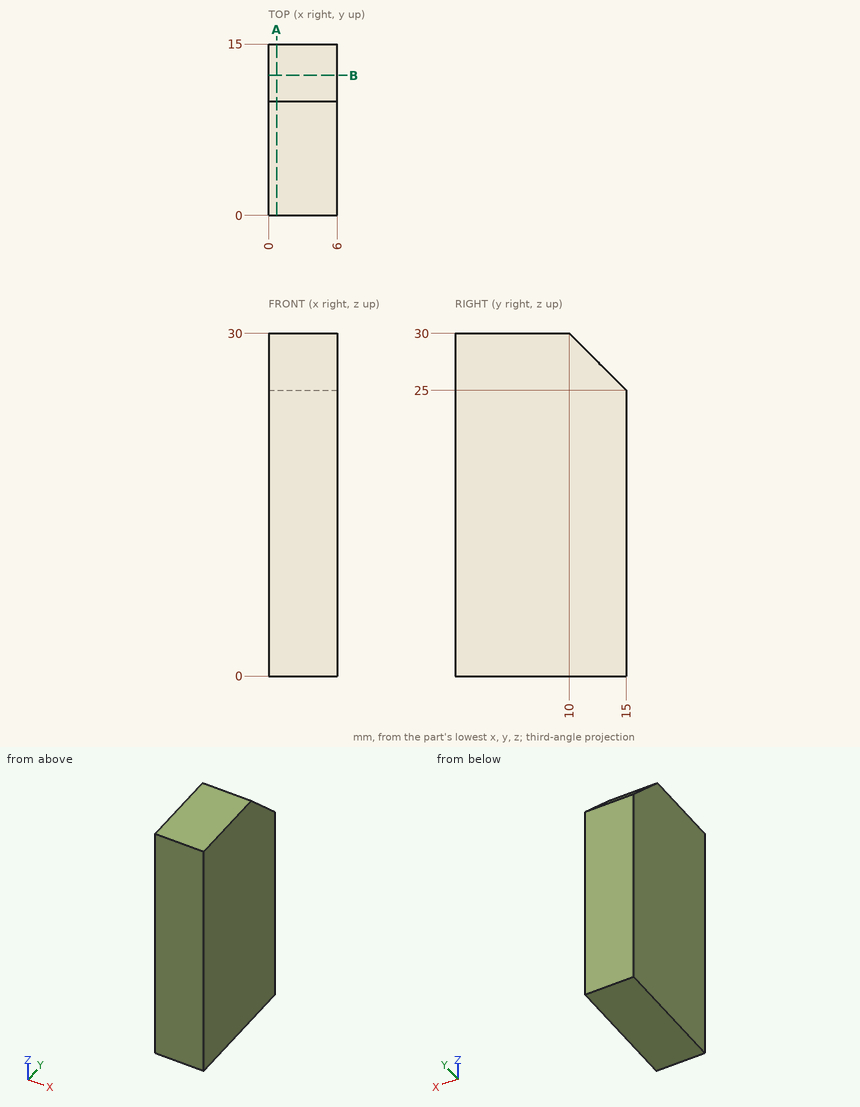
Drawing for the job (mm, zero at the part's lowest x, y, z). Round coordinates to 2 decimals unless told otherwise and drop trailing zeros. Loops run counter-clockwise (first coordinate to the right, second up) from the corner with the lowest first, then second, coordinate; pieces in that order, holes last. Notation, with made-up numbers: (24, 86) - (53, 86) arc R18 cw to (53, 98) - close; hole circle Ø11 at (-5, -14). An arc over 180 degrees is marked (long way). Write each question's results on one line, items separated by ' | '.
(1) Wall check: L1, parallel to Z at x = 5.3, y = 12; L2, parallel to Y at x = 1.35, z = 25.5; L3, parallel to Y at x = 2.2, z = 27. Give the ranges that are in metal, low to high.
Answer below:
L1: z = 0 to 28 | L2: y = 0 to 14.5 | L3: y = 0 to 13
(2) Pin check, flat tip, straight feed: pin 1 (6 mm diameter, centred on y = 10, z = 12.5, fed in from -X). Stop position of the tip, or through.
Answer below:
pin 1: stops at x = 0
(3) Saw through at A-A, the plane x = 0.7. List the corners of the cut face in (y, z).
Answer below:
outline: (0, 0) - (15, 0) - (15, 25) - (10, 30) - (0, 30) - close
(4) Saw through at B-B, the plane y = 12.25. List the corners of the cut face in (x, z).
Answer below:
outline: (0, 0) - (6, 0) - (6, 27.75) - (0, 27.75) - close
